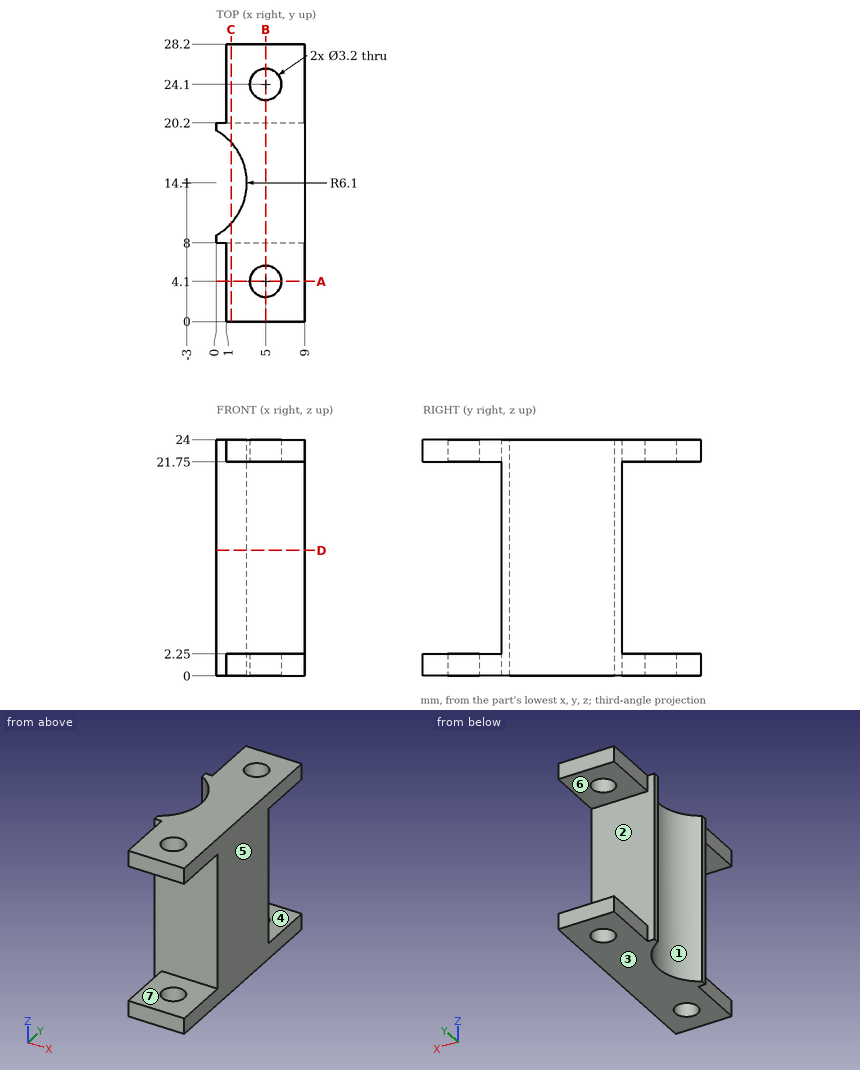
The figure shows three views and two pictorial views of one solid part (mm, origin at its lowest corner). Answer the questions. A direction names the side the tool comes from. Give positions to 0.01 mm unless a question says otherwise; leave off trailing zeros. Order: outer loops, then holes, each group sorted by start corner. A loop starts at its lowest first (then second) coordinate and runs counter-clockwise, first axis right, second up. Notation, with made-up numbers: (49, -39) - (64, -39) arc R20 ccw to (64, -22) - close; hole circle Ø10 at (14.25, -38). An arc over 180 degrees is marked (long way). Answer as CSV lines item,"result".
Q1. Each of these flat-tipped pins is pushed along its axis until it touches: pin 1 Ø3 at (x, z) = (3.5, 9.5) entering from -Y; pin 2 Ø1.1 at (y, z) = (2, 23) entering from -X; pin 3 Ø4.5 at (x, z) = (6.5, 16) entering from +Y. Where does it stop, or does it pass through?
Answer key:
pin 1,"stops at y = 8"
pin 2,"stops at x = 1"
pin 3,"stops at y = 20.2"
Q2. A cutting plane is placed at B-B, the plane x = 5. Determine the outline of the cut face in (y, z).
Answer key:
outline,"(0, 0) - (2.5, 0) - (2.5, 2.25) - (0, 2.25) - close; (0, 21.75) - (2.5, 21.75) - (2.5, 24) - (0, 24) - close; (5.7, 0) - (22.5, 0) - (22.5, 2.25) - (20.2, 2.25) - (20.2, 21.75) - (22.5, 21.75) - (22.5, 24) - (5.7, 24) - (5.7, 21.75) - (8, 21.75) - (8, 2.25) - (5.7, 2.25) - close; (25.7, 0) - (28.2, 0) - (28.2, 2.25) - (25.7, 2.25) - close; (25.7, 21.75) - (28.2, 21.75) - (28.2, 24) - (25.7, 24) - close"
Q3. A cutting plane is placed at C-C, the plane x = 1.5. Determine the outline of the cut face in (y, z), and give its area (3 significant figures).
Answer key:
outline,"(0, 0) - (9.98, 0) - (9.98, 24) - (0, 24) - (0, 21.75) - (8, 21.75) - (8, 2.25) - (0, 2.25) - close; (18.22, 0) - (28.2, 0) - (28.2, 2.25) - (20.2, 2.25) - (20.2, 21.75) - (28.2, 21.75) - (28.2, 24) - (18.22, 24) - close"
area,"167 mm^2"
Q4. A cutting plane is placed at A-A, the plane y = 4.1. Determine the outline of the cut face in (x, z).
Answer key:
outline,"(1, 0) - (3.4, 0) - (3.4, 2.25) - (1, 2.25) - close; (1, 21.75) - (3.4, 21.75) - (3.4, 24) - (1, 24) - close; (6.6, 0) - (9, 0) - (9, 2.25) - (6.6, 2.25) - close; (6.6, 21.75) - (9, 21.75) - (9, 24) - (6.6, 24) - close"
Q5. Straight lines are drawn through the part: L1, parallel to Y at x = 5, z = 22.3; L2, parallel to X at y = 4.1, z = 1.3; L3, parallel to Z at x = 8, y = 23. For each, find the intervals that lie inside material, in ascending order.
Answer key:
L1,"y = 0 to 2.5, 5.7 to 22.5, 25.7 to 28.2"
L2,"x = 1 to 3.4, 6.6 to 9"
L3,"z = 0 to 2.25, 21.75 to 24"
Q6. Which of the six approach directions +Z, -Z, +X, -X, +Y, -Y give full straight-line access (tool end or side, diameter ignored) to the marked faces 5, 6 and 7?
Answer key:
face 5,"+Z, -Z, +X, +Y, -Y"
face 6,"+X, -X, +Y"
face 7,"+X, -X, -Y"
Q7. A cutting plane is placed at D-D, the plane z = 12.75. Determine the outline of the cut face in (x, y).
Answer key:
outline,"(0, 8) - (9, 8) - (9, 20.2) - (0, 20.2) - (0, 19.41) arc R6.1 cw to (0, 8.79) - close"
Q8. Determine the mould class of the marked faces 1, 2, 3 and 4 for opening direction Z: pulls with the +Z half, pulls with the -Z half, needs draft (parallel to the pull), parting line crosses it, or undercut.
Answer key:
face 1,"needs draft"
face 2,"undercut"
face 3,"pulls with the -Z half"
face 4,"undercut"
